Build history of the part. All positions in model axes, mm. Coordinates: 2 decimals unless noted, no trailing zeros. Write each loop counter-clockwise with the first axis right and the second up, starting at its lowest first coordinate (ties: lowest second). Pieces come first, ordered by that corner, then holes.
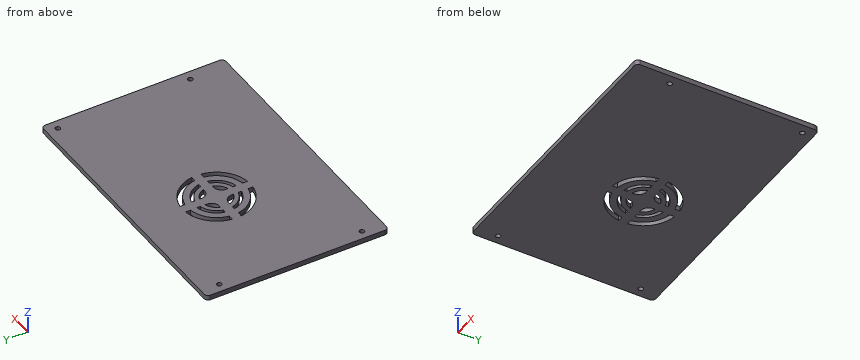
```python
from build123d import *

# Parameters (mm, degrees)
SKETCH1_W           = 174.752
SKETCH1_H           = 115.824
SKETCH1_R           = 1.5494
BOSS_EXTRUDE2_DEPTH = 3.175
FILLET2_R           = 2.54


with BuildPart() as part:
    # Sketch1 → Boss-Extrude2 (new body)
    with BuildSketch(Plane.XY):
        with Locations((87.376, 57.912)):
            Rectangle(SKETCH1_W, SKETCH1_H)
        with BuildLine():
            Line((51.201113755, 62.918740671), (54.351132043, 62.918740671))
            ThreePointArc((54.351132043, 62.918740671), (59.551059271, 52.693059261), (69.776740685, 47.493132041))
            Line((69.776740685, 47.493132041), (69.776740685, 44.343113753))
            ThreePointArc((69.776740685, 44.343113753), (57.34663836, 50.48863835), (51.201113755, 62.918740671))
        make_face(mode=Mode.SUBTRACT)
        with BuildLine():
            Line((58.47906711, 62.918740671), (60.598040919, 62.918740671))
            ThreePointArc((60.598040919, 62.918740671), (63.888250287, 57.030250277), (69.776740685, 53.740040915))
            Line((69.776740685, 53.740040915), (69.776740685, 51.621067107))
            ThreePointArc((69.776740685, 51.621067107), (62.424741229, 55.566741219), (58.47906711, 62.918740671))
        make_face(mode=Mode.SUBTRACT)
        with BuildLine():
            ThreePointArc((69.776740685, 56.70280403), (65.908807914, 59.050807904), (63.560804035, 62.918740671))
            Line((63.560804035, 62.918740671), (64.696740685, 62.918740671))
            ThreePointArc((64.696740685, 62.918740671), (68.288843133, 61.43084312), (69.776740685, 57.838740671))
            Line((69.776740685, 57.838740671), (69.776740685, 56.70280403))
        make_face(mode=Mode.SUBTRACT)
        with BuildLine():
            ThreePointArc((75.511259315, 47.493132041), (85.736940729, 52.693059261), (90.936867957, 62.918740671))
            Line((90.936867957, 62.918740671), (94.086886245, 62.918740671))
            ThreePointArc((94.086886245, 62.918740671), (87.94136164, 50.48863835), (75.511259315, 44.343113753))
            Line((75.511259315, 44.343113753), (75.511259315, 47.493132041))
        make_face(mode=Mode.SUBTRACT)
        with BuildLine():
            ThreePointArc((75.511259315, 53.740040915), (81.399749713, 57.030250277), (84.689959081, 62.918740671))
            Line((84.689959081, 62.918740671), (86.80893289, 62.918740671))
            ThreePointArc((86.80893289, 62.918740671), (82.863258771, 55.566741219), (75.511259315, 51.621067107))
            Line((75.511259315, 51.621067107), (75.511259315, 53.740040915))
        make_face(mode=Mode.SUBTRACT)
        with BuildLine():
            Line((80.591259315, 62.918740671), (81.727195965, 62.918740671))
            ThreePointArc((81.727195965, 62.918740671), (79.379192086, 59.050807904), (75.511259315, 56.70280403))
            Line((75.511259315, 56.70280403), (75.511259315, 57.838740671))
            ThreePointArc((75.511259315, 57.838740671), (76.999156867, 61.43084312), (80.591259315, 62.918740671))
        make_face(mode=Mode.SUBTRACT)
        with BuildLine():
            Line((64.696740685, 68.653259329), (63.560804035, 68.653259329))
            ThreePointArc((63.560804035, 68.653259329), (65.908807914, 72.521192096), (69.776740685, 74.86919597))
            Line((69.776740685, 74.86919597), (69.776740685, 73.733259329))
            ThreePointArc((69.776740685, 73.733259329), (68.288843133, 70.14115688), (64.696740685, 68.653259329))
        make_face(mode=Mode.SUBTRACT)
        with BuildLine():
            Line((69.776740685, 79.950932893), (69.776740685, 77.831959085))
            ThreePointArc((69.776740685, 77.831959085), (63.888250287, 74.541749723), (60.598040919, 68.653259329))
            Line((60.598040919, 68.653259329), (58.47906711, 68.653259329))
            ThreePointArc((58.47906711, 68.653259329), (62.424741229, 76.005258781), (69.776740685, 79.950932893))
        make_face(mode=Mode.SUBTRACT)
        with BuildLine():
            ThreePointArc((69.776740685, 84.078867959), (59.551059271, 78.878940739), (54.351132043, 68.653259329))
            Line((54.351132043, 68.653259329), (51.201113755, 68.653259329))
            ThreePointArc((51.201113755, 68.653259329), (57.34663836, 81.08336165), (69.776740685, 87.228886247))
            Line((69.776740685, 87.228886247), (69.776740685, 84.078867959))
        make_face(mode=Mode.SUBTRACT)
        with BuildLine():
            Line((75.511259315, 73.733259329), (75.511259315, 74.86919597))
            ThreePointArc((75.511259315, 74.86919597), (79.379192086, 72.521192096), (81.727195965, 68.653259329))
            Line((81.727195965, 68.653259329), (80.591259315, 68.653259329))
            ThreePointArc((80.591259315, 68.653259329), (76.999156867, 70.14115688), (75.511259315, 73.733259329))
        make_face(mode=Mode.SUBTRACT)
        with BuildLine():
            Line((86.80893289, 68.653259329), (84.689959081, 68.653259329))
            ThreePointArc((84.689959081, 68.653259329), (81.399749713, 74.541749723), (75.511259315, 77.831959085))
            Line((75.511259315, 77.831959085), (75.511259315, 79.950932893))
            ThreePointArc((75.511259315, 79.950932893), (82.863258771, 76.005258781), (86.80893289, 68.653259329))
        make_face(mode=Mode.SUBTRACT)
        with BuildLine():
            ThreePointArc((90.936867957, 68.653259329), (85.736940729, 78.878940739), (75.511259315, 84.078867959))
            Line((75.511259315, 84.078867959), (75.511259315, 87.228886247))
            ThreePointArc((75.511259315, 87.228886247), (87.94136164, 81.08336165), (94.086886245, 68.653259329))
            Line((94.086886245, 68.653259329), (90.936867957, 68.653259329))
        make_face(mode=Mode.SUBTRACT)
        with Locations((5.6642, 13.6144)):
            Circle(SKETCH1_R, mode=Mode.SUBTRACT)
        with Locations((168.6814, 24.6888)):
            Circle(SKETCH1_R, mode=Mode.SUBTRACT)
        with Locations((5.6642, 104.267)):
            Circle(SKETCH1_R, mode=Mode.SUBTRACT)
        with Locations((168.6814, 108.966)):
            Circle(SKETCH1_R, mode=Mode.SUBTRACT)
    extrude(amount=BOSS_EXTRUDE2_DEPTH)

    # Fillet2
    fillet2_edges = [part.edges().sort_by_distance(p)[0] for p in [
        (174.752, 0, 1.5875),
        (0, 0, 1.5875),
        (0, 115.824, 1.5875),
        (174.752, 115.824, 1.5875),
    ]]
    fillet(fillet2_edges, radius=FILLET2_R)


solid = part.part
```
1. Saw through at A-A on x = 66.5. List the corners of the cut face in (y, z) (3 decimals), plus the area to 3 significant figures.
Computed values:
outline: (0, 0) - (45.043, 0) - (45.043, 3.175) - (0, 3.175) - close; (48.319, 0) - (52.705, 0) - (52.705, 3.175) - (48.319, 3.175) - close; (55.035, 0) - (58.507, 0) - (58.507, 3.175) - (55.035, 3.175) - close; (62.588, 0) - (68.984, 0) - (68.984, 3.175) - (62.588, 3.175) - close; (73.065, 0) - (76.537, 0) - (76.537, 3.175) - (73.065, 3.175) - close; (78.867, 0) - (83.253, 0) - (83.253, 3.175) - (78.867, 3.175) - close; (86.529, 0) - (115.824, 0) - (115.824, 3.175) - (86.529, 3.175) - close
area: 306 mm2
2. Saw through at B-B on z = 2.3. State how many separate pieces and enclosed holes the cut face has, plus the area to 3 significant figures.
Computed values:
separate pieces: 1
enclosed holes: 16
area: 19,700 mm2
3. Probe line 1 along X through (y, z) = (46, 1.1); line 2 along X through (y, z) = (24.5, 0.25); line 3 along X through (y, z) = (47, 2.6). List the from-to ranges inside material, lowest first.
Computed values:
line 1: x = 0 to 63.9, 69.78 to 75.51, 81.39 to 174.75
line 2: x = 0 to 167.14, 170.22 to 174.75
line 3: x = 0 to 61.92, 69.78 to 75.51, 83.37 to 174.75
